Can you work these out from the model? Positions are in its coordinate system, mm. A direction names the side the tool comes from. Give positions to 0.01 mm unless a question says otherwise; leave off trailing zeros. Write each loop counter-clockwise with the first axis right and the second up, starting at its lowest first coordinate (ties: lowest second). Pieces come first, ordered by that corner, then holes.
1. Suppose I cut it at D-D (x = -33.5). Please give me the cut outline in (y, z), and give its area (3 significant figures).
2. On a 3-axis mill with a long thin cutter (end or side, diameter ignored), from which of +Z, -Z, +X, -X, +Y, -Y can I reach the whole of each face in a straight line? I mean faces 4 (the cylindrical face through (3, 0, 55)), 5 (the cylindrical face through (-35.87, -1.76, -39.96)), 6 (the cylindrical face through (-13.542, -41.375, -46.112)). Say none if no direction works.
3. Suppose I cut it at C-C (x = -14). Give the number of separate pieces and of enclosed holes in the cut face, and give its area (3 significant figures).
4. If I drill on probe 1 along Y at (x, z) = (-13.5, 0); probe 2 along X at (y, z) = (-13.5, 36.5); probe 3 along X at (y, z) = (-43, 58.5), over which ranges is the centre line in solid material (lowest first)?
5. Thinking about a two-plate mould opening in Z: for faces 1 (the cylindrical face through (-5.161, 58.436, 58.237)), 2 (the flat face through (6.5, 57, 1)), 3 (the flat face through (0, 35.9, -11.5)), which applies, pulls with the +Z half, pulls with the -Z half, needs draft (parallel to the pull), parting line crosses it, or undercut?
6. I'm going to push flat-ended pins straight in: pin 1 (19.5 mm diameter, centred on y = 40.66, z = 40.66, fed in from -X); pin 2 (6.5 mm diameter, centred on y = 51.27, z = 51.27, fed in from +X); pin 3 (8 mm diameter, centred on x = -29, y = -10.5, fed in from +Z); pin 4 (8 mm diameter, centred on x = -27.5, z = -21, fed in from -Y). Where does each tip first touch, or does it pass through?
7. Suppose I cut it at A-A (y = 0). Please give me the cut outline in (x, z).
```python
from build123d import *

# Parameters (mm, degrees)
SKETCH_3_OUTSIDE_W           = 214.814
SKETCH_3_OUTSIDE_H           = 214.814
SKETCH_3_OUTSIDE_W_2         = 130
SKETCH_3_OUTSIDE_H_2         = 130
CUT_EXTRUDE_1_DEPTH          = 121.222710001
SKETCH_4_R                   = 4
CUT_EXTRUDE_2_DEPTH          = 106.61249926
HOLE_WIZARD_M6_1_D           = 11
HOLE_WIZARD_M6_1_CBORE_D     = 17
HOLE_WIZARD_M6_1_CBORE_DEPTH = 17
PATTERN_CIRCULAR_1_COUNT     = 4


with BuildPart() as part:
    # 草图2 → 旋转1 (revolve)
    with BuildSketch(Plane.XY, mode=Mode.PRIVATE) as revolve_1_sk:
        Polygon((0, 37.5), (0, 55), (6.5, 55), (6.5, 82.5), (-16.5, 82.5), (-16.5, 47.25), (-45.5, 47.25), (-45.5, 40), (-26.5, 40), (-26.5, 37.5), align=None)
    revolve(revolve_1_sk.sketch.rotate(Axis((0, 0, 0), (1, 0, 0)), 90), axis=Axis((0, 0, 0), (1, 0, 0)))

    # 草图3 outside → 切除-拉伸1 (cut, through all)
    with BuildSketch(Plane.ZY.offset(16.5)):
        Rectangle(SKETCH_3_OUTSIDE_W, SKETCH_3_OUTSIDE_H)
        Rectangle(SKETCH_3_OUTSIDE_W_2, SKETCH_3_OUTSIDE_H_2, mode=Mode.SUBTRACT)
    extrude(amount=-CUT_EXTRUDE_1_DEPTH, mode=Mode.SUBTRACT)

    # 草图4 → 切除-拉伸2 (cut, through all)
    with BuildSketch(Plane.ZY.offset(45.5)):
        with Locations((-51.265241636, 51.265241636)):
            Circle(SKETCH_4_R)
        with Locations((51.265241636, 51.265241636)):
            Circle(SKETCH_4_R)
        with Locations((51.265241636, -51.265241636)):
            Circle(SKETCH_4_R)
        with Locations((-51.265241636, -51.265241636)):
            Circle(SKETCH_4_R)
    extrude(amount=-CUT_EXTRUDE_2_DEPTH, mode=Mode.SUBTRACT)

    # M6 六角头螺栓的柱形沉头孔1 (through all)
    with Locations(Plane(origin=(6.5, 0, 0), x_dir=(0, 0, -1), z_dir=(1, 0, 0))):
        with Locations((40.658639918, 40.658639918)):
            hole_wizard_m6_1 = CounterBoreHole(HOLE_WIZARD_M6_1_D / 2, HOLE_WIZARD_M6_1_CBORE_D / 2, HOLE_WIZARD_M6_1_CBORE_DEPTH)

    # 阵列(圆周)1: M6 六角头螺栓的柱形沉头孔1 ×4 about axis
    pattern_circular_1_axis = Axis((0, 0, 0), (1, 0, 0))
    for i in range(1, PATTERN_CIRCULAR_1_COUNT):
        add(hole_wizard_m6_1.rotate(pattern_circular_1_axis, i * 360 / PATTERN_CIRCULAR_1_COUNT), mode=Mode.SUBTRACT)


solid = part.part
```
Checks:
1. outline: circle Ø94.5 at (0, 0); hole circle Ø80 at (0, 0)
1. area: 1,990 mm2
2. face 4: +X
2. face 5: -X
2. face 6: +X, -X
3. separate pieces: 1
3. enclosed holes: 9
3. area: 11,500 mm2
4. probe 1: y = -65 to -37.5, 37.5 to 65
4. probe 2: x = -26.5 to 0
4. probe 3: x = -16.5 to 6.5
5. face 1: pulls with the +Z half
5. face 2: needs draft
5. face 3: undercut
6. pin 1: stops at x = -16.5
6. pin 2: passes through
6. pin 3: stops at z = 46.8
6. pin 4: stops at y = -44.09
7. outline: (-45.5, -47.25) - (-16.5, -47.25) - (-16.5, -65) - (6.5, -65) - (6.5, -55) - (0, -55) - (0, -37.5) - (-26.5, -37.5) - (-26.5, -40) - (-45.5, -40) - close; (-45.5, 40) - (-26.5, 40) - (-26.5, 37.5) - (0, 37.5) - (0, 55) - (6.5, 55) - (6.5, 65) - (-16.5, 65) - (-16.5, 47.25) - (-45.5, 47.25) - close
